Answer from the drawing. Dimensions are ordinates in mm from the lowest x, y and z of the part. Round coordinates to 2 decimals unless told otherwise and drop trailing zeros. Write each loop counter-clockwise with the first axis right and the second up, starting at its lowest first coordinate (ties: lowest second). Pieces come first, ordered by that corner, then holes.
1. Find section D-D (y = 32.5). Write down the section's boundary in (x, z), and give its area (3 significant figures).
2. Determine the mould class of the marked faces 1, 2 and 3 for opening direction X: pulls with the +X half, pulls with the -X half, needs draft (parallel to the pull), parting line crosses it, or undercut.
3. Flat-ended cylindrical pins translate along their axes: pin 1 Ø1.5 at (x, z) = (18.5, 17) entering from +Y; pin 2 Ø6 at (x, z) = (23, 19.5) entering from -Y; pin 3 Ø3 at (x, z) = (27, 26.5) entering from -Y; pin 4 Ø6 at (x, z) = (14.5, 40.5) entering from -Y. Find the tip coordinate at first contact, or state that the pin passes through.
4. Straight lines are drawn through the part: probe 1 along X at (y, z) = (19, 16); probe 2 along X at (y, z) = (15.5, 48.5). For each, find the intervals that lie inside material, in ascending order.
5. Find section A-A (x = 19.05). Write down the section's boundary in (y, z), and give its area (3 significant figures).
6. Find section C-C (y = 28.5). Write down the section's boundary in (x, z) (1 decimal).
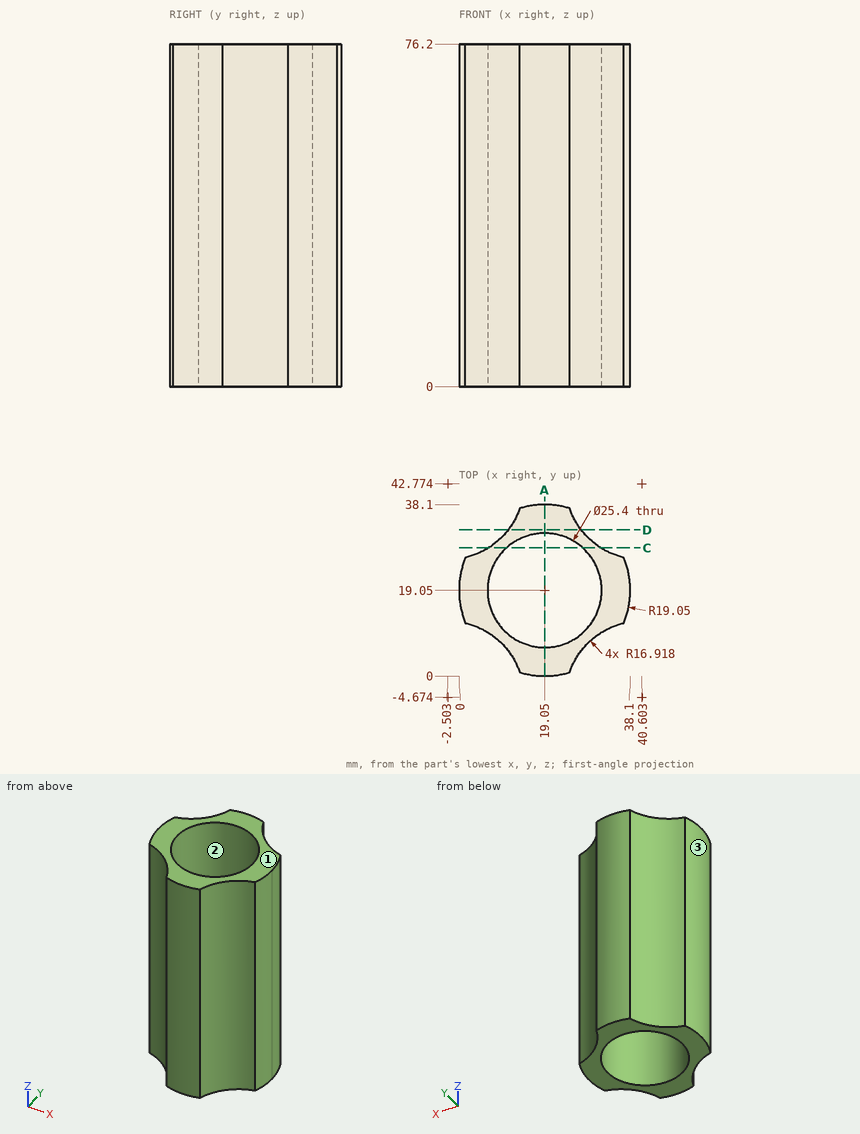
Worked answers:
1. outline: (10.94, 0) - (27.16, 0) - (27.16, 76.2) - (10.94, 76.2) - close
1. area: 1,240 mm2
2. face 1: needs draft
2. face 2: undercut
2. face 3: pulls with the -X half
3. pin 1: stops at y = 38.1
3. pin 2: stops at y = 0.02
3. pin 3: stops at y = 2.95
3. pin 4: stops at y = 0.06
4. probe 1: x = 0 to 6.35, 31.75 to 38.1
4. probe 2: x = 0.33 to 6.86, 31.24 to 37.77
5. outline: (0, 0) - (6.35, 0) - (6.35, 76.2) - (0, 76.2) - close; (31.75, 0) - (38.1, 0) - (38.1, 76.2) - (31.75, 76.2) - close
5. area: 968 mm2
6. outline: (6.6, 0) - (10.6, 0) - (10.6, 76.2) - (6.6, 76.2) - close; (27.5, 0) - (31.5, 0) - (31.5, 76.2) - (27.5, 76.2) - close
